Part print with two shaded views. Sizes in mm from the minimum x, y, z corner. A direction names the side the tool comes from. Coordinates: 2 decimals unless noted, no trailing zeros. Write each loop counter-clockwise with the first axis right and the second up, starting at its lowest first coordinate (ties: lowest second). Pieces come first, ordered by that corner, then holes. Notation, with made-up numbers: (17.5, -7) - (35.5, -7) arc R22 cw to (35.5, 14) - close; hole circle Ø7 at (52, 78.5). An arc over 180 degrees is marked (long way). Answer in a Markdown table with one row per item. Add a question column.
Q1. Band-saw the part on D-D (y = 10.5). List the corners of the cut face in (x, z), and give its area (3 significant figures).
Q2. Drill centre lines: line 1 along X through (y, z) = (1, 4); line 2 along X through (y, z) = (0.3, 4); line 3 along X through (y, z) = (6.25, 6.5). Where is each one in solid material? Low to high. Write a range as from..to.
Q3. Two-plate mould, pull along X, no slides. Class the marked faces 1, 2 and 3: +X half, -X half, draft (parallel to the pull), parting line (faces both ways), or undercut.
Q4. Pin check, flat tips, straight feed: pin 1 (0.7 mm diameter, centred on x = 20.5, y = 0.5, fed in from +Z); pin 2 (6 mm diameter, centred on y = 7, z = 9, fed in from +X); pin 3 (2.5 mm diameter, centred on x = 3, z = 4, fed in from -Y); pin 4 (3 mm diameter, centred on x = 3, z = 4.5, fed in from +Y). Stop position of each tip, or through.
Q5. Band-saw the part on A-A (y = 8.75). List the corners of the cut face in (x, z), and give its area (3 significant figures).
Q6. Band-saw the part on C-C (z = 8.5). List the corners of the cut face in (x, y).
Q7. 3-axis set-ups, long thin cutter, end or side, ignore diameter. For the marked faces 4, 5, 6, 7 and 8: which of +Z, -Z, +X, -X, +Y, -Y reach the whole face in a straight line?
Q8. Band-saw the part on B-B (x = 2.75). List the corners of the cut face in (y, z).
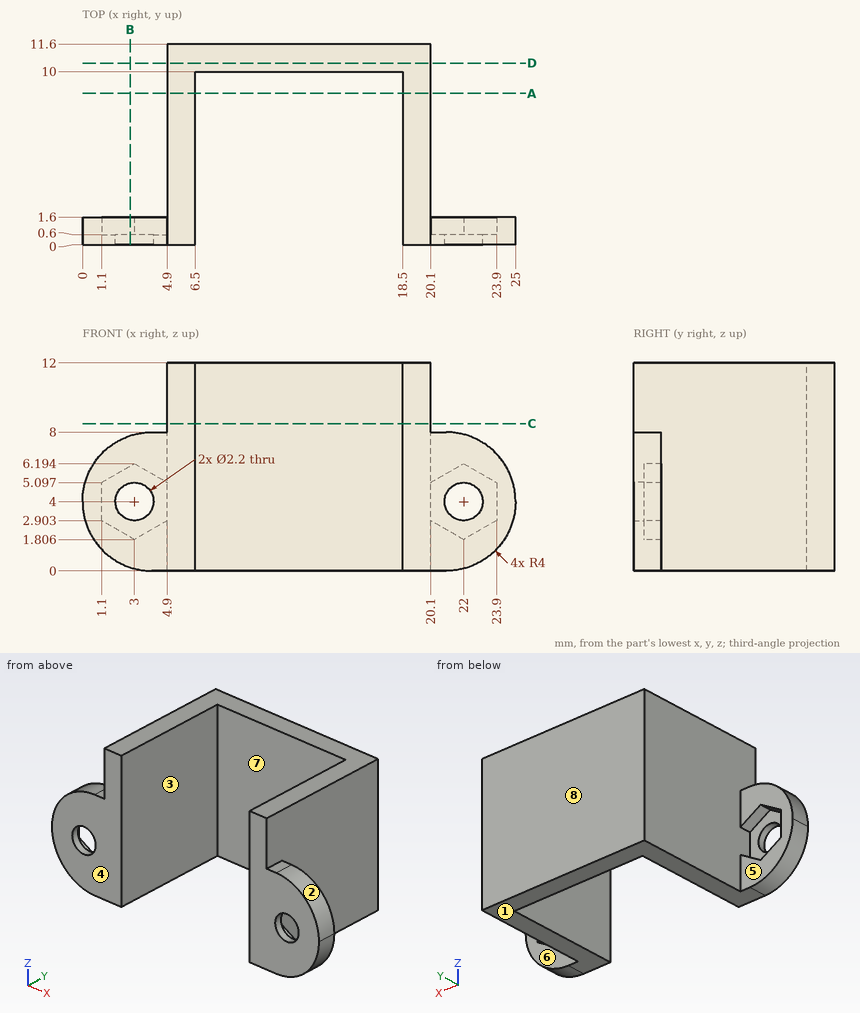
Checked values:
| question | item | result |
|---|---|---|
| 1 | outline | (4.9, 0) - (20.1, 0) - (20.1, 12) - (4.9, 12) - close |
| 1 | area | 182 mm² |
| 2 | line 1 | x = 0..1.1, 4.9..6.5, 18.5..20.1, 23.9..25 |
| 2 | line 2 | x = 0..1.9, 4.1..6.5, 18.5..20.9, 23.1..25 |
| 2 | line 3 | x = 4.9..6.5, 18.5..20.1 |
| 3 | face 1 | draft |
| 3 | face 2 | +X half |
| 3 | face 3 | undercut |
| 4 | pin 1 | stops at z = 8 |
| 4 | pin 2 | stops at x = 20.1 |
| 4 | pin 3 | stops at y = 0 |
| 4 | pin 4 | stops at y = 1.6 |
| 5 | outline | (4.9, 0) - (6.5, 0) - (6.5, 12) - (4.9, 12) - close; (18.5, 0) - (20.1, 0) - (20.1, 12) - (18.5, 12) - close |
| 5 | area | 38.4 mm² |
| 6 | outline | (4.9, 0) - (6.5, 0) - (6.5, 10) - (18.5, 10) - (18.5, 0) - (20.1, 0) - (20.1, 11.6) - (4.9, 11.6) - close |
| 7 | face 4 | +Z, -Z, +X, -X, -Y |
| 7 | face 5 | +Z, -Z, -X, +Y |
| 7 | face 6 | +Z, -Z, +X, +Y |
| 7 | face 7 | +Z, -Z, -Y |
| 7 | face 8 | +Z, -Z, +X, -X, +Y |
| 8 | outline | (0, 0.2) - (1.6, 0.2) - (1.6, 1.95) - (0.6, 1.95) - (0.6, 2.93) - (0, 2.93) - close; (0, 5.07) - (0.6, 5.07) - (0.6, 6.05) - (1.6, 6.05) - (1.6, 7.8) - (0, 7.8) - close |
